Could you check a few things on this model? Use its own coordinates, in mm. A direction names the side the tool comes from. Round coordinates to 2 decimals unless told otherwise and drop trailing zeros. Order: outer loops, then holes, each group sorted by start corner. A loop starts at its lowest first (then second) coordinate and runs counter-clockwise, first axis right, second up. Notation, with made-up numbers: (58, 37.25) - (112, 37.25) arc R28 ccw to (112, 60.25) - close; hole circle Ø4 at (-12.75, -37.5). An arc over 180 degrees is marked (long way). Return JSON: item names as keys, results as strings. Group by question number.
Autodesk Inventor part; units mm, degrees
ref_plane "YZ Plane" through (0, 0, 0) normal (1, 0, 0) x (0, 1, 0)
ref_plane "XZ Plane" through (0, 0, 0) normal (0, 1, 0) x (-1, 0, 0)
ref_plane "XY Plane" through (0, 0, 0) normal (0, 0, 1) x (1, 0, 0)
sketch "Esboço1" plane through (0, 0, 0) normal (0, 0, 1) x (1, 0, 0)
  line L0 (-18, 25.5) -> (338, 25.5)
  line L1 (340, 23.5) -> (340, -8.5)
  line L2 (-20, -8.5) -> (-20, 23.5)
  circle A0 centre (0, 0) radius 5.995 construction
  circle A1 centre (320, 0) radius 5.995 construction
  line L3 (6, -10.5) -> (18.7017, 11.5)
  line L4 (6, -10.5) -> (31.4034, -10.5) construction
  line L5 (18.7017, 11.5) -> (161.7689, 11.5)
  line L6 (160, 31.3493) -> (160, -25.519) construction
  line L7 (314, -10.5) -> (301.2983, 11.5)
  line L8 (301.2983, 11.5) -> (161.7689, 11.5)
  line L9 (-18, 25.5) -> (-20, 23.5)
  line L10 (-20, -8.5) -> (-18, -10.5)
  line L11 (338, 25.5) -> (340, 23.5)
  line L12 (338, -10.5) -> (340, -8.5)
  line L13 (338, -10.5) -> (314, -10.5)
  line L14 (6, -10.5) -> (-18, -10.5)
  circle A2 centre (0, 0) radius 6
  circle A3 centre (320, 0) radius 6
  point P0 (340, -10.5)
  point P1 (340, 25.5)
  point P2 (-20, -10.5)
  point P3 (-20, 25.5)
  dimension "d0" = 36
  dimension "d2" = 2
  dimension "d3" = 2
  dimension "d4" = 2
  dimension "d5" = 2
  dimension "d6" = 2
  dimension "d7" = 2
  dimension "d8" = 2
  dimension "d9" = 2
  dimension "d10" = 12
  dimension "d11" = 12
  dimension "d14" = 120
  dimension "d15" = 14
  dimension "d16" = 24
extrude "Extrusão1" add sketch "Esboço1" against normal blind 9.52
properties part number "EsbarrosCarro"
1) For faces 4 (the flat face through (162, 11.5, -5)), 5 (the flat face through (-20, 7, -5)), which set-ups out of +Z, -Z, +X, -X, +Y, -Y let a thin tool reach every point of the face, with its end or its side?
2) I want a section at C-C, the plane y = 0. List the corners of the cut face in (x, z) for me.
3) I want a section at D-D, the plane x = 109. List the corners of the cut face in (y, z) for me.
4) Will these pins go through, and if not, where does the flat tip stop? pin 1 (11 mm diameter, centred on x = 320, y = 0, fed in from +Z); pin 2 (5 mm diameter, centred on x = 85, z = -6.5, fed in from -Y).
5) I want a section at B-B, the plane x = 0. List the corners of the cut face in (y, z) for me.
6) If I drill on line 1 along Y through (x, z) = (320, -5.25); line 2 along X through (y, z) = (3, -6.25); line 3 along Y through (x, z) = (200.5, -8.5), over which ranges is the centre line in solid material (lowest first)? Write a range as from..to.
7) We'd pull the mould along Y, two halves only. Please class faces 1 (the flat face through (307.738, 0.346, -4.693)), 2 (the flat face through (158, 25.5, -5)), 3 (the cylindrical face through (-6, 0, -5)): +Y half, -Y half, draft (parallel to the pull), parting line (faces both ways), or undercut.
8) I want a section at A-A, the plane z = -1.5. List the corners of the cut face in (x, y) for me.
Outcome:
{
 "1": {"face 4": "+Z, -Z, -Y", "face 5": "+Z, -Z, -X, +Y, -Y"},
 "2": {"outline": "(-20, -9.52) - (-6, -9.52) - (-6, 0) - (-20, 0) - close; (6, -9.52) - (12.06, -9.52) - (12.06, 0) - (6, 0) - close; (307.94, -9.52) - (314, -9.52) - (314, 0) - (307.94, 0) - close; (326, -9.52) - (340, -9.52) - (340, 0) - (326, 0) - close"},
 "3": {"outline": "(11.5, -9.52) - (25.5, -9.52) - (25.5, 0) - (11.5, 0) - close"},
 "4": {"pin 1": "through", "pin 2": "y = 11.5"},
 "5": {"outline": "(-10.5, -9.52) - (-6, -9.52) - (-6, 0) - (-10.5, 0) - close; (6, -9.52) - (25.5, -9.52) - (25.5, 0) - (6, 0) - close"},
 "6": {"line 1": "-10.5..-6, 6..25.5", "line 2": "-20..-5.2, 5.2..13.79, 306.21..314.8, 325.2..340", "line 3": "11.5..25.5"},
 "7": {"face 1": "-Y half", "face 2": "+Y half", "face 3": "undercut"},
 "8": {"outline": "(-20, -8.5) - (-18, -10.5) - (6, -10.5) - (18.7, 11.5) - (301.3, 11.5) - (314, -10.5) - (338, -10.5) - (340, -8.5) - (340, 23.5) - (338, 25.5) - (-18, 25.5) - (-20, 23.5) - close; hole circle Ø12 at (0, 0); hole circle Ø12 at (320, 0)"}
}
